```python
from build123d import *

# Parameters (mm, degrees)
F1_DEPTH  = 78.6
F4_DEPTH  = 72.6
F5_W      = 18
F5_H      = 72.6
F6_DEPTH  = 5
F8_DEPTH  = 5
F10_DEPTH = 5
F11_R     = 5
F12_R     = 2
F13_W     = 10.3
F13_H     = 3
F14_DEPTH = 42.5
F16_R     = 1.95
F17_DEPTH = 4
F18_SIZE  = 2
F19_R     = 2


with BuildPart() as f1:
    # F0 (on Front) → F1 (new body)
    with BuildSketch(Plane.XZ):
        Polygon((-50, 0), (0, 0), (0, 60), (-15, 60), (-50, 30), align=None)
    extrude(amount=F1_DEPTH)

    # F3 (on offset) → F4 (cut)
    with BuildSketch(Plane.XZ.offset(3)):
        Polygon((-47, 4), (0, 4), (0, 33.5), (-3, 33.5), (-3, 54), (-17.3902277714, 54), (-47, 28.6201952326), align=None)
    extrude(amount=F4_DEPTH, mode=Mode.SUBTRACT)

    # F5 (on face) → F6 (cut)
    with BuildSketch(Plane(origin=(0, 0, 0), x_dir=(1, 0, 0), z_dir=(0, 0, -1))):
        with Locations((-9, 39.3)):
            Rectangle(F5_W, F5_H)
    extrude(amount=-F6_DEPTH, mode=Mode.SUBTRACT)

    # F7 (on Front) → F8 (cut)
    with BuildSketch(Plane.XZ):
        with BuildLine():
            Line((-6.5, 24), (0, 24))
            Line((0, 24), (0, 28))
            Line((0, 28), (-6.5, 28))
            ThreePointArc((-6.5, 28), (-7.5606601718, 27.5606601718), (-8, 26.5))
            Line((-8, 26.5), (-8, 25.5))
            ThreePointArc((-8, 25.5), (-7.5606601718, 24.4393398282), (-6.5, 24))
        make_face()
    extrude(amount=F8_DEPTH, mode=Mode.SUBTRACT)

    # F9 (on face) → F10 (cut)
    with BuildSketch(Plane.XZ.offset(78.6)):
        with BuildLine():
            Line((-8, 24), (0, 24))
            Line((0, 24), (0, 31))
            Line((0, 31), (-8, 31))
            ThreePointArc((-8, 31), (-10.1213203436, 30.1213203436), (-11, 28))
            Line((-11, 28), (-11, 27))
            ThreePointArc((-11, 27), (-10.1213203436, 24.8786796564), (-8, 24))
        make_face()
    extrude(amount=-F10_DEPTH, mode=Mode.SUBTRACT)

    # F11
    f11_edges = [f1.edges().sort_by_distance(p)[0] for p in [
        (-15, -39.3, 60),
        (-50, -39.3, 30),
        (-50, -39.3, 0),
    ]]
    fillet(f11_edges, radius=F11_R)

    # F12
    f12_edges = [f1.edges().sort_by_distance(p)[0] for p in [
        (-32.329147, 0, 45.146446),
        (-32.329147, -78.6, 45.146446),
        (-22.5, 0, 0),
        (-22.5, -78.6, 0),
        (-50, 0, 16.350163),
        (-49.542564, 0, 29.789609),
        (-48.535534, 0, 1.464466),
        (-14.885111, 0, 59.689425),
        (-6.57519, 0, 60),
        (-48.535534, -78.6, 1.464466),
        (-50, -78.6, 16.350163),
        (-49.542564, -78.6, 29.789609),
        (-14.885111, -78.6, 59.689425),
        (-6.57519, -78.6, 60),
        (-10.195114, -3, 54),
        (-32.195114, -3, 41.310098),
        (-47, -3, 16.310098),
        (-47, -75.6, 16.310098),
        (-32.195114, -75.6, 41.310098),
        (-10.195114, -75.6, 54),
        (-17.390228, -39.3, 54),
        (-47, -39.3, 28.620195),
    ]]
    fillet(f12_edges, radius=F12_R)

    # F13 (on face) → F14 (join)
    with BuildSketch(Plane.YZ.offset(-47)):
        with Locations((-8.15, 5.5)):
            Rectangle(F13_W, F13_H)
        with Locations((-70.45, 5.5)):
            Rectangle(F13_W, F13_H)
    extrude(amount=F14_DEPTH)

    # F16 (on offset) → F17 (join)
    with BuildSketch(Plane.XY.offset(4)):
        with Locations((-10.5, -9.3)):
            Circle(F16_R)
        with Locations((-10.5, -69.3)):
            Circle(F16_R)
    extrude(amount=-F17_DEPTH)

    # F18
    f18_edges = [f1.edges().sort_by_distance(p)[0] for p in [
        (-3, -39.3, 33.5),
    ]]
    chamfer(f18_edges, length=F18_SIZE)

    # F19
    f19_edges = [f1.edges().sort_by_distance(p)[0] for p in [
        (-47, -9.15, 7),
        (-47, -13.3, 5.5),
        (-47, -69.45, 7),
        (-47, -65.3, 5.5),
        (-24.75, -75.6, 7),
        (-24.75, -3, 7),
        (-46.414214, -3.585786, 7),
        (-32.5, -13.3, 4),
        (-32.5, -65.3, 4),
        (-46.414214, -75.014214, 7),
    ]]
    fillet(f19_edges, radius=F19_R)


solid = f1.part
```
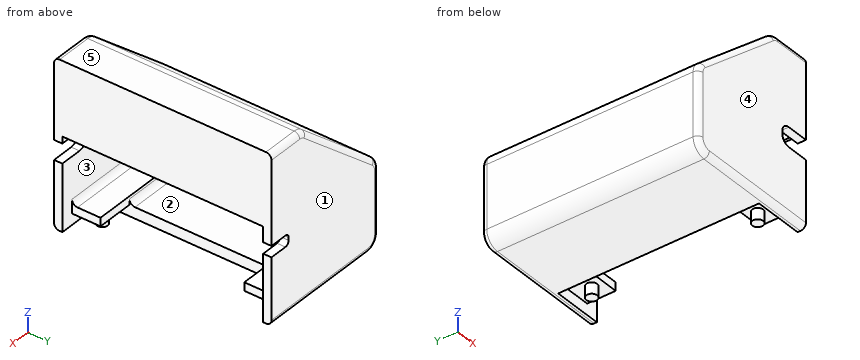
Verification items for the finished model (mm, model axes). Face numbers are marked on the shaded views. A direction names the side the tool comes from. Round coordinates to 2 decimals unless told otherwise and drop trailing zeros. Write each loop counter-clockwise with the first axis right and the second up, starting at its lowest first coordinate (ties: lowest second). Pieces come first, ordered by that corner, then holes. Notation, with made-up numbers: (47, 2.25) - (75, 2.25) arc R19 cw to (75, 27.25) - close; hole circle Ø9 at (77, 80.25). An arc over 180 degrees is marked (long way). Answer as a JSON object with one key per item and string values. Group by question number.
Q1. Section check B-B, the plane z = 21.5. Enter the section's corners in (x, y).
Q2. Section check A-A, the plane y = -30.5. Enter the section's corners in (x, z).
Q3. Go/stop test with flat-tipped pins: pin 1 Ø0.9 at (x, y) = (-4.5, -77.5) entering from -Z; pin 2 Ø6.5 at (x, y) = (-33, -70) entering from +Z; pin 3 Ø6.5 at (y, z) = (-44.5, 2) entering from +X. Record where each tip stops, or that it passes through.
Q4. Section check C-C, the plane y = -9.3. Enter the section's corners in (x, z).
Q5. Mould release check, pull along Y, two halves, no side actions. Record for the marked faces 3, 4 and 5: released by +Y, released by -Y, zero draft, split by the parting line, or undercut.
Q6. Tool access check on the marked faces 1 and 2. Record the directions out of +Z, -Z, +X, -X, +Y, -Y that give a thin tool (end or side, any length) a straight path to the whole face; none if there is none.
Q7. Thickness scan on line 1 (Y direction, x = -19, z = 37); line 2 (X direction, y = -11, z = 24.5); line 3 (Z direction, x = -12.5, y = -52). Record the ranges inside material, lowest first.
Found:
{
 "1": {"outline": "(-50, -76.6) arc R2 ccw to (-48, -78.6) - (0, -78.6) - (0, -75.6) - (-45, -75.6) arc R2 cw to (-47, -73.6) - (-47, -5) arc R2 cw to (-45, -3) - (0, -3) - (0, 0) - (-48, 0) arc R2 ccw to (-50, -2) - close"},
 "2": {"outline": "(-50, 5) arc R5 ccw to (-45, 0) - (-18, 0) - (-18, 4) - (-47, 4) - (-47, 27.7) arc R2 cw to (-46.3, 29.22) - (-17.95, 53.52) arc R2 cw to (-16.65, 54) - (-3, 54) - (-3, 35.5) - (-1, 33.5) - (0, 33.5) - (0, 60) - (-13.15, 60) arc R5 ccw to (-16.4, 58.8) - (-48.25, 31.5) arc R5 ccw to (-50, 27.7) - close"},
 "3": {"pin 1": "stops at z = 0.05", "pin 2": "stops at z = 47.36", "pin 3": "stops at x = -18"},
 "4": {"outline": "(-50, 5) arc R5 ccw to (-45, 0) - (-18, 0) - (-18, 4) - (-12.45, 4) - (-12.45, 0) - (-8.55, 0) - (-8.55, 4) - (-4.5, 4) - (-4.5, 7) - (-45, 7) arc R2 cw to (-47, 9) - (-47, 27.7) arc R2 cw to (-46.3, 29.22) - (-17.95, 53.52) arc R2 cw to (-16.65, 54) - (-3, 54) - (-3, 35.5) - (-1, 33.5) - (0, 33.5) - (0, 60) - (-13.15, 60) arc R5 ccw to (-16.4, 58.8) - (-48.25, 31.5) arc R5 ccw to (-50, 27.7) - close"},
 "5": {"face 3": "undercut", "face 4": "released by -Y", "face 5": "zero draft"},
 "6": {"face 1": "+Z, -Z, +X, -X, +Y", "face 2": "+X"},
 "7": {"line 1": "y = -78.6 to -75.6, -3 to 0", "line 2": "x = -50 to -47", "line 3": "z = 54 to 60"}
}
